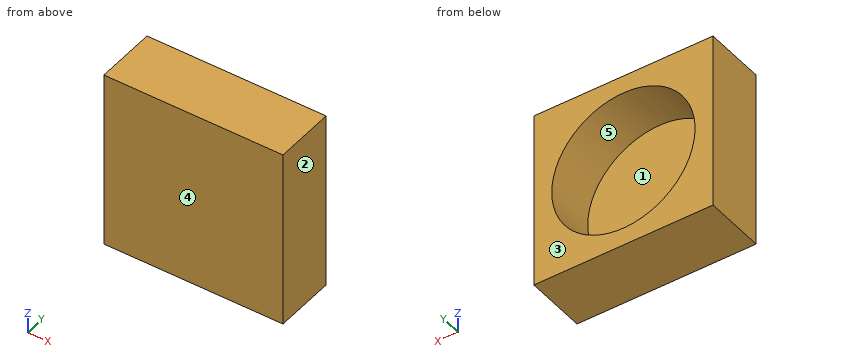
Autodesk Inventor part; units mm, degrees
ref_plane "YZ Plane" through (0, 0, 0) normal (1, 0, 0) x (0, 1, 0)
ref_plane "XZ Plane" through (0, 0, 0) normal (0, 1, 0) x (-1, 0, 0)
ref_plane "XY Plane" through (0, 0, 0) normal (0, 0, 1) x (1, 0, 0)
sketch "Esquisse1" plane through (0, 0, 0) normal (0, 1, 0) x (-1, 0, 0)
  line L0 (0, 0) -> (350, 0)
  line L1 (350, 0) -> (350, -350)
  line L2 (350, -350) -> (0, -350)
  line L3 (0, -350) -> (0, 0)
  dimension "d0" = 350
  dimension "d1" = 350
extrude "Extrusion1" add sketch "Esquisse1" along normal blind 120
sketch "Esquisse2" plane through (0, 120, 0) normal (0, 1, 0) x (1, 0, 0)
  line L0 (0, 350) -> (-350, 350)
  line L1 (-350, 350) -> (-350, 0)
  circle A0 centre (-175, 175) radius 140
  point P0 (0, 0)
  dimension "d4" = 175
  dimension "d5" = 175
  dimension "d6" = 280
extrude "Extrusion2" cut sketch "Esquisse2" against normal blind 100
Can you work these out from the model? Positions are in its coordinate system, mm. Face numbers are marked on the shaded views. A direction names the side the tool comes from. Round coordinates to 2 decimals unless told otherwise and drop trailing zeros. Write each loop counter-clockwise with the first axis right and the second up, starting at its lowest first coordinate (ties: lowest second). Pieces come first, ordered by that corner, then holes. Notation, with made-up numbers: (43, -3) -> (57, -3) arc R16 cw to (57, 11) -> close; hole circle Ø8 at (1, -10.75). An arc over 180 degrees is marked (long way). One line per question, with ' | ' between items. Start each with the question number.
1) If we mould it in two halves opening along Y, with no side actions, what happens to the marked faces 3, 4 and 5? For each: released by +Y, released by -Y, zero draft, split by the parting line, or undercut.
2) Suppose I cut it at C-C on x = -175. Write out the boundary of the cut face in (y, z).
3) I'm going to push a flat-ended pin straight in: P1, Ø12, axis at x = -75, z = -144, coming from the +Y side. Where does the tip first touch, or does it pass through?
4) Suppose I cut it at B-B on z = -175. Write out the boundary of the cut face in (x, y), then the cut area to 3 significant figures.
5) On a 3-axis mill with a long thin cutter (end or side, diameter ignored), from which of +Z, -Z, +X, -X, +Y, -Y can I reach the whole of each face in a straight line? I mean the marked faces 1 and 2. Say none if no direction works.
6) I need wall thicknesses on line 1 (X direction, y = 59, z = -175); line 2 (Z direction, x = -143, y = 38.5). Which ranges of each line are inside material? Lowest first, please. Write a range as [from, to].
7) Suppose I cut it at A-A on y = 111. Write out the boundary of the cut face in (x, z).
Return value:
1) face 3: released by +Y | face 4: released by -Y | face 5: zero draft
2) outline: (0, -350) -> (120, -350) -> (120, -315) -> (20, -315) -> (20, -35) -> (120, -35) -> (120, 0) -> (0, 0) -> close
3) P1: stops at y = 20
4) outline: (-350, 0) -> (0, 0) -> (0, 120) -> (-35, 120) -> (-35, 20) -> (-315, 20) -> (-315, 120) -> (-350, 120) -> close | area: 14,000 mm2
5) face 1: +Y | face 2: +Z, -Z, +X, +Y, -Y
6) line 1: x = [-350, -315], [-35, 0] | line 2: z = [-350, -311.29], [-38.71, 0]
7) outline: (-350, -350) -> (0, -350) -> (0, 0) -> (-350, 0) -> close; hole circle Ø280 at (-175, -175)
